Build history of the part. All positions in model axes, mm. Face numbers are marked on the shaded views. Round coordinates to 2 decimals unless told otherwise and drop trailing zeros. Write each loop counter-clockwise with the first axis right and the second up, starting at its lowest first coordinate (ties: lowest second). Pieces come first, ordered by that corner, then holes.
from build123d import *

# Parameters (mm, degrees)
SKETCH_1_W         = 7
SKETCH_1_H         = 20
EXTRUDE_1_DEPTH    = 56.57
SKETCH_2_W         = 15
SKETCH_2_H         = 12
EXTRUDE_2_DEPTH    = 6
HOLE_WIZARD_M4_1_D = 3.3


with BuildPart() as part:
    # 草图1 → 凸台-拉伸1 (new, symmetric)
    with BuildSketch(Plane(origin=(0, 0, 0), x_dir=(0, 0, -1), z_dir=(1, 0, 0))):
        Rectangle(SKETCH_1_W, SKETCH_1_H)
    extrude(amount=EXTRUDE_1_DEPTH, both=True)

    # 草图2 → 凸台-拉伸2 (add)
    with BuildSketch(Plane(origin=(0, 0, -3.5), x_dir=(-1, 0, 0), z_dir=(0, 0, -1))):
        with Locations((-34.07, 4)):
            Rectangle(SKETCH_2_W, SKETCH_2_H)
    extrude_2 = extrude(amount=EXTRUDE_2_DEPTH)

    # 镜向1: 凸台-拉伸2 across plane
    add(extrude_2.mirror(Plane(origin=(0, 0, 0), x_dir=(0, 0, 1), z_dir=(1, 0, 0))))

    # M4 螺纹孔1 (through all)
    with Locations(Plane(origin=(0, -2, 0), x_dir=(-1, 0, 0), z_dir=(0, -1, 0))):
        with Locations((34, 6.5), (-34, 6.5)):
            Hole(HOLE_WIZARD_M4_1_D / 2)


solid = part.part
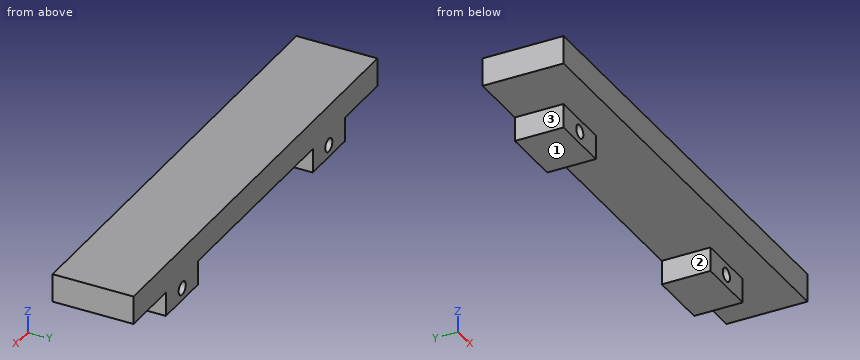
1) Pin check, flat tips, straight feed: pin 1 Ø2.5 at (x, z) = (-34, -6.5) entering from +Y; pin 2 Ø3 at (y, z) = (7.5, -8) entering from -X; pin 3 Ø10 at (x, y) = (1, -3) entering from -Z; pin 4 Ø5 at (x, z) = (-34.5, -8) entering from -Y. Stop position of each tip, or through.
Results:
pin 1: passes through
pin 2: stops at x = -41.57
pin 3: stops at z = -3.5
pin 4: stops at y = -2
2) Wall check: L1, parallel to X at y = 1.75, z = -6.5; L2, parallel to Z at x = 34, y = 5.75; L3, parallel to X at y = 1, z = -7.5. Give the ranges that are in metal, low to high.
Results:
L1: x = -41.57 to -35.65, -32.35 to -26.57, 26.57 to 32.35, 35.65 to 41.57
L2: z = -9.5 to -8.15, -4.85 to 3.5
L3: x = -41.57 to -35.31, -32.69 to -26.57, 26.57 to 32.69, 35.31 to 41.57
3) Slice it at A-A (x = 34). Write the cut outline in (y, z), plus the area to 3 significant figures.
Results:
outline: (-10, -3.5) - (-2, -3.5) - (-2, -4.85) - (10, -4.85) - (10, 3.5) - (-10, 3.5) - close; (-2, -9.5) - (10, -9.5) - (10, -8.15) - (-2, -8.15) - close
area: 172 mm2
4) Slice it at B-B (y = 0.25). Write the cut outline in (x, z).
Results:
outline: (-56.57, -3.5) - (-41.57, -3.5) - (-41.57, -9.5) - (-26.57, -9.5) - (-26.57, -3.5) - (26.57, -3.5) - (26.57, -9.5) - (41.57, -9.5) - (41.57, -3.5) - (56.57, -3.5) - (56.57, 3.5) - (-56.57, 3.5) - close; hole circle Ø3.3 at (-34, -6.5); hole circle Ø3.3 at (34, -6.5)
5) Mould opens along X. For the marked faces 1, 2 and 3 say: released by +X, released by -X, zero draft, split by the parting line, or undercut.
Results:
face 1: zero draft
face 2: undercut
face 3: released by -X
6) Slice it at D-D (x = -48). Write the cut outline in (y, z).
Results:
outline: (-10, -3.5) - (10, -3.5) - (10, 3.5) - (-10, 3.5) - close
7) Slice it at C-C (z = -6.5). Write the cut outline in (x, y).
Results:
outline: (-41.57, -2) - (-35.65, -2) - (-35.65, 10) - (-41.57, 10) - close; (-32.35, -2) - (-26.57, -2) - (-26.57, 10) - (-32.35, 10) - close; (26.57, -2) - (32.35, -2) - (32.35, 10) - (26.57, 10) - close; (35.65, -2) - (41.57, -2) - (41.57, 10) - (35.65, 10) - close
